```python
from build123d import *

# Parameters (mm, degrees)
F1_DEPTH = 5
F3_DEPTH = 5
F5_D     = 5.5


with BuildPart() as f1:
    # F0 (on Top) → F1 (new body)
    with BuildSketch(Plane.XY):
        with BuildLine():
            Line((-14, 11.313708499), (-14, -11.313708499))
            ThreePointArc((-14, -11.313708499), (0, -18), (14, -11.313708499))
            Line((14, -11.313708499), (14, 11.313708499))
            ThreePointArc((14, 11.313708499), (0, 18), (-14, 11.313708499))
        make_face()
    extrude(amount=F1_DEPTH)

    # F2 (on face) → F3 (join)
    with BuildSketch(Plane.XY.offset(5)):
        with BuildLine():
            Line((-5, 17.2916164658), (-5, 0))
            ThreePointArc((-5, 0), (0, -5), (5, 0))
            Line((5, 0), (5, 17.2916164658))
            ThreePointArc((5, 17.2916164658), (0, 18), (-5, 17.2916164658))
        make_face()
    extrude(amount=F3_DEPTH)

    # F5 (through all)
    with Locations(Plane(origin=(0, 0, 0), x_dir=(1, 0, 0), z_dir=(0, 0, -1))):
        with Locations((0, 0)):
            Hole(F5_D / 2)


solid = f1.part
```
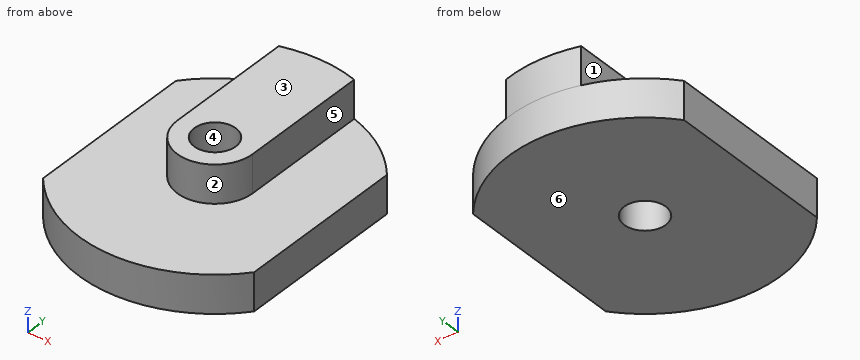
Read the model definition and answer for the solid it produces. Units are mm, in the model's axes. Face numbers are marked on the shaded views. A direction names the side the tool comes from. Round coordinates to 2 decimals unless told otherwise and drop trailing zeros. Loops run counter-clockwise (first coordinate to the right, second up) from the corner with the lowest first, then second, coordinate; pieces in that order, holes last. Notation, with made-up numbers: (85.5, 71) -> (89.5, 71) arc R18 ccw to (89.5, 77) -> close; hole circle Ø2 at (-38.5, -12.5). An arc over 180 degrees is marked (long way). One line per item, written item: value.
1) For the marked faces 1, 2 and 3, determine the directions among +Z, -Z, +X, -X, +Y, -Y from which every point of the face is accessible in a straight line to the end or side of a thin tool.
Answer list:
face 1: +Z, -X, +Y, -Y
face 2: +Z, -Y
face 3: +Z, +X, -X, +Y, -Y
2) The mould has two halves that part along X. Classify the marked faces 4, 5 and 6: pulls with the +X half, pulls with the -X half, needs draft (parallel to the pull), parting line crosses it, or undercut.
Answer list:
face 4: undercut
face 5: pulls with the +X half
face 6: needs draft
3) A cutting plane is placed at C-C (y = 9). Determine the outline of the cut face in (x, z), and give its area (3 significant figures).
Answer list:
outline: (-14, 0) -> (14, 0) -> (14, 5) -> (5, 5) -> (5, 10) -> (-5, 10) -> (-5, 5) -> (-14, 5) -> close
area: 190 mm²
4) Consider L1, parallel to Y at x = 0, z = 5.5; L2, parallel to Y at x = 0, z = 3.5; L3, parallel to Z at x = -11.75, y = -12.5. Determine where each line is inside the solid, lowest interval first. Write a range as [from, to].
Answer list:
L1: y = [-5, -2.75], [2.75, 18]
L2: y = [-18, -2.75], [2.75, 18]
L3: z = [0, 5]
5) A cutting plane is placed at A-A (x = 0). Determine the outline of the cut face in (y, z).
Answer list:
outline: (-18, 0) -> (-2.75, 0) -> (-2.75, 10) -> (-5, 10) -> (-5, 5) -> (-18, 5) -> close; (2.75, 0) -> (18, 0) -> (18, 10) -> (2.75, 10) -> close
6) A cutting plane is placed at D-D (z = 7.5). Determine the outline of the cut face in (x, y).
Answer list:
outline: (-5, 0) arc R5 ccw to (5, 0) -> (5, 17.29) arc R18 ccw to (-5, 17.29) -> close; hole circle Ø5.5 at (0, 0)
7) A cutting plane is placed at B-B (z = 0.5). Determine the outline of the cut face in (x, y), and give its area (3 significant figures).
Answer list:
outline: (-14, -11.31) arc R18 ccw to (14, -11.31) -> (14, 11.31) arc R18 ccw to (-14, 11.31) -> close; hole circle Ø5.5 at (0, 0)
area: 870 mm²
8) Flat-ended cylindrical pins translate along their axes: P1, Ø1.5, axis at y = 5, z = 8, coming from the -X side; P2, Ø1.5, axis at x = 6, y = 3.5, coming from the +Z side; P3, Ø5, axis at x = 10.5, z = 2, coming from the -Y side. Find the tip coordinate at first contact, or state that the pin passes through.
Answer list:
P1: stops at x = -5
P2: stops at z = 5
P3: stops at y = -16.12
